```python
from build123d import *

# Parameters (mm, degrees)
ESQUISSE1_W                                        = 165
ESQUISSE1_H                                        = 52.75
BOSS_EXTRU_1_DEPTH                                 = 5
BOSS_EXTRU_2_DEPTH                                 = 41
ESQUISSE3_W                                        = 149.5
ESQUISSE3_H                                        = 5
ENL_V_MAT_EXTRU_1_DEPTH                            = 36
D_GAGEMENT_M31_D                                   = 3.4
D_GAGEMENT_M31_DEPTH                               = 6
D_GAGEMENT_M31_TIP                                 = 1.021463052
CHAMBRAGE_POUR_VIS_SIX_PANS_CREUX_2_COUNT          = 2
CHAMBRAGE_POUR_VIS_SIX_PANS_CREUX_2_PITCH          = 28.7
SKETCH7_W                                          = 35.36
SKETCH7_H                                          = 5
BOSS_EXTRUDE1_DEPTH                                = 9.25
CHAMBRAGE_POUR_VIS_T_TE_HEXAGONALE_M61_D           = 7
CHAMBRAGE_POUR_VIS_T_TE_HEXAGONALE_M61_CBORE_D     = 14.547
CHAMBRAGE_POUR_VIS_T_TE_HEXAGONALE_M61_CBORE_DEPTH = 4


with BuildPart() as part:
    # Esquisse1 → Boss.-Extru.1 (new body)
    with BuildSketch(Plane.XY):
        with Locations((51.592169311, -5.600810811)):
            Rectangle(ESQUISSE1_W, ESQUISSE1_H)
    extrude(amount=BOSS_EXTRU_1_DEPTH)

    # Esquisse2 → Boss.-Extru.2 (add)
    with BuildSketch(Plane.XY.offset(5)):
        Polygon((-30.907830689, 20.774189189), (-23.157830689, 20.774189189), (-23.157830689, -2.975810811), (126.342169311, -2.975810811), (126.342169311, 20.774189189), (134.092169311, 20.774189189), (134.092169311, -31.975810811), (126.342169311, -31.975810811), (126.342169311, -7.975810811), (-23.157830689, -7.975810811), (-23.157830689, -31.975810811), (-30.907830689, -31.975810811), align=None)
    extrude(amount=BOSS_EXTRU_2_DEPTH)

    # Esquisse3 → Enlèv. mat.-Extru.1 (cut)
    with BuildSketch(Plane.XY.offset(46)):
        with Locations((51.592169311, -5.475810811)):
            Rectangle(ESQUISSE3_W, ESQUISSE3_H)
    extrude(amount=-ENL_V_MAT_EXTRU_1_DEPTH, mode=Mode.SUBTRACT)

    # Dégagement M31
    with Locations(Plane.XY.offset(46)):
        with Locations((-27.220932929, 16.149189189), (130.405271551, 16.149189189), (130.405271551, -27.350810811), (-27.220932929, -27.350810811)):
            Hole(D_GAGEMENT_M31_D / 2, depth=D_GAGEMENT_M31_DEPTH)
            with Locations((0, 0, -(D_GAGEMENT_M31_DEPTH + D_GAGEMENT_M31_TIP / 2))):  # 118° drill point
                Cone(0, D_GAGEMENT_M31_D / 2, D_GAGEMENT_M31_TIP, mode=Mode.SUBTRACT)

    # Sketch5 → Chambrage pour vis à six pans creux M2.51 (revolve, cut)
    with BuildSketch(Plane(origin=(51.592169311, 13.774189189, 5), x_dir=(0, -1, 0), z_dir=(1, 0, 0))):
        Polygon((0, 0), (0, 5), (1.55, 5), (1.55, 2.9), (2.75, 2.9), (2.75, 0.025), (2.775, 0), align=None)
    chambrage_pour_vis_six_pans_creux_m2_5 = revolve(axis=Axis((51.592169311, 13.774189189, 11.35), (0, 0, -1)), mode=Mode.SUBTRACT)

    # Chambrage pour vis _ six pans creux  2: Chambrage pour vis à six pans creux M2.51 ×2
    with Locations(*[(0, -i * CHAMBRAGE_POUR_VIS_SIX_PANS_CREUX_2_PITCH, 0) for i in range(1, CHAMBRAGE_POUR_VIS_SIX_PANS_CREUX_2_COUNT)]):
        add(chambrage_pour_vis_six_pans_creux_m2_5, mode=Mode.SUBTRACT)

    # Sketch7 → Boss-Extrude1 (add)
    with BuildSketch(Plane.XZ.offset(31.975810811)):
        with Locations((51.592169311, 2.5)):
            Rectangle(SKETCH7_W, SKETCH7_H)
    extrude(amount=BOSS_EXTRUDE1_DEPTH)

    # Chambrage pour vis à tête hexagonale M61 (through all)
    with Locations(Plane.XY.offset(5)):
        with Locations((51.592169311, -31.275810811)):
            CounterBoreHole(CHAMBRAGE_POUR_VIS_T_TE_HEXAGONALE_M61_D / 2, CHAMBRAGE_POUR_VIS_T_TE_HEXAGONALE_M61_CBORE_D / 2, CHAMBRAGE_POUR_VIS_T_TE_HEXAGONALE_M61_CBORE_DEPTH)


solid = part.part
```
Geometry check sheet. Reference: the model listing, model coordinates, mm. A direction names the side the tool comes from. Coordinates: 2 decimals unless noted, no trailing zeros. Write each loop counter-clockwise with the first axis right and the second up, starting at its lowest first coordinate (ties: lowest second). Pieces come first, ordered by that corner, then holes. Notation, with made-up numbers: M -37,45.25 L 9,45.25 A26 cw 9,84.25 Z; hole C -20.5,24 d11. An arc over 180 degrees is marked long. One line per item, written item: value. Start each with the question number.
(1) Sectioned sample at B-B, the plane x = 7. Enter the section's corners in (y, z).
(2) Sectioned sample at A-A, the plane z = 27.5. Enter the section's corners in (x, y), and give its area (3 significant figures).
(3) Release check for a two-part mould opening along X. For faces 1 (the face through (-10, -31.976, 4)), 2 (the face through (33.912, -37, 2)), 3 (the face through (50.055, -14.724, 1.065)) record: released by +X, released by -X, zero draft, split by the parting line, or undercut.
(4) Sectioned sample at C-C, the plane y = -5.5. Enter the section's corners in (x, z).
(5) Scan lines: line 1 along X through (y, z) = (-5, 30.5); line 2 along Z through (x, y) = (60.5, 17.5); line 3 along Z through (x, y) = (13.5, -5). Record each from-to range of solid material in increasing order. Write a range as [from, to].
(6) Tool access check on faces 4 (the face through (51, 9, 5)), 5 (the face through (69.272, -37, 2)), 6 (the face through (51, -5, 10)), 7 (the face through (49.27, 12.3, 3.56)). Record the directions out of +Z, -Z, +X, -X, +Y, -Y that give a thin tool (end or side, any length) a straight path to the whole face; none if there is none.
(7) Depth check by flat-ended pin: pin 1 (12 mm diameter, centred on x = 46.5, y = 6.5, fed in from +Z); pin 2 (1 mm diameter, centred on x = 68.5, z = 8.5, fed in from -Y); pin 3 (5.5 mm diameter, centred on x = 72, y = -6, fed in from +Z). Enter the tip coordinate at first touch or a pass-through.
Filled sheet:
1. outline: M -31.98,0 L 20.77,0 L 20.77,5 L -2.98,5 L -2.98,10 L -7.98,10 L -7.98,5 L -31.98,5 Z
2. outline: M -30.91,-31.98 L -23.16,-31.98 L -23.16,20.77 L -30.91,20.77 Z; M 126.34,-31.98 L 134.09,-31.98 L 134.09,20.77 L 126.34,20.77 Z
2. area: 818 mm²
3. face 1: zero draft
3. face 2: released by -X
3. face 3: undercut
4. outline: M -30.91,0 L 134.09,0 L 134.09,46 L 126.34,46 L 126.34,10 L -23.16,10 L -23.16,46 L -30.91,46 Z
5. line 1: [-30.91, -23.16], [126.34, 134.09]
5. line 2: [0, 5]
5. line 3: [0, 10]
6. face 4: +Z, +Y
6. face 5: +Z, -Z, +X, -Y
6. face 6: +Z, +Y, -Y
6. face 7: +Z
7. pin 1: z = 5
7. pin 2: y = -7.98
7. pin 3: z = 10
